from build123d import *

# Parameters (mm, degrees)
SKETCH1_W           = 44.45
SKETCH1_H           = 19.05
BOSS_EXTRUDE1_DEPTH = 12.7
SKETCH2_W           = 7.62
SKETCH2_H           = 16.51
CUT_EXTRUDE1_DEPTH  = 12.7
FILLET1_R           = 1.27
FILLET2_R           = 1.27
SKETCH3_R           = 1.6256
CUT_EXTRUDE2_DEPTH  = 12.7
SKETCH4_R           = 1.651
CUT_EXTRUDE3_DEPTH  = 12.7


with BuildPart() as part:
    # Sketch1 → Boss-Extrude1 (new body)
    with BuildSketch(Plane.XY):
        Rectangle(SKETCH1_W, SKETCH1_H)
    extrude(amount=BOSS_EXTRUDE1_DEPTH)

    # Sketch2 → Cut-Extrude1 (cut)
    with BuildSketch(Plane.XY.offset(12.7)):
        with Locations((-18.415, 1.27)):
            Rectangle(SKETCH2_W, SKETCH2_H)
        with Locations((18.415, 1.27)):
            Rectangle(SKETCH2_W, SKETCH2_H)
    extrude(amount=-CUT_EXTRUDE1_DEPTH, mode=Mode.SUBTRACT)

    # Fillet1
    fillet1_edges = [part.edges().sort_by_distance(p)[0] for p in [
        (-14.605, -6.985, 6.35),
    ]]
    fillet(fillet1_edges, radius=FILLET1_R)

    # Fillet2
    fillet2_edges = [part.edges().sort_by_distance(p)[0] for p in [
        (14.605, -6.985, 6.35),
    ]]
    fillet(fillet2_edges, radius=FILLET2_R)

    # Sketch3 → Cut-Extrude2 (cut)
    with BuildSketch(Plane(origin=(0, 0, 0), x_dir=(-1, 0, 0), z_dir=(0, 0, -1))):
        with Locations((-9.525, 5.715)):
            Circle(SKETCH3_R)
        with Locations((9.525, 5.715)):
            Circle(SKETCH3_R)
    extrude(amount=-CUT_EXTRUDE2_DEPTH, mode=Mode.SUBTRACT)

    # Sketch4 → Cut-Extrude3 (cut)
    with BuildSketch(Plane(origin=(0, -6.985, 0), x_dir=(1, 0, 0), z_dir=(0, 1, 0))):
        with Locations(Location((19.05, -6.35, 0), (0, 0, 180))):
            Circle(SKETCH4_R)
        with Locations(Location((-19.05, -6.4262, 0), (0, 0, 180))):
            Circle(SKETCH4_R)
    extrude(amount=-CUT_EXTRUDE3_DEPTH, mode=Mode.SUBTRACT)


solid = part.part
The model under review builds one solid part; all positions refer to its coordinate system, in mm. A direction names the side the tool comes from. Round coordinates to 2 decimals unless told otherwise and drop trailing zeros. Order: outer loops, then holes, each group sorted by start corner. A loop starts at its lowest first (then second) coordinate and runs counter-clockwise, first axis right, second up. Notation, with made-up numbers: (49.25, -35.75) -> (99.25, -35.75) arc R27 ccw to (99.25, -9.75) -> close; hole circle Ø8 at (21, -33). An arc over 180 degrees is marked (long way). Write item = value, one per line. Start each with the question number.
Item 1: Consider section C-C on z = 5.75. Write out the cut boundary in (x, y) (3 decimals).
Item 2: Mouldability with a two-part tool opening along X and no side actions: class faces 1 (the face through (14.605, 2, 6)), 2 (the face through (-17.4, -8.2, 6.5)), 3 (the face through (18, -6.985, 8)) as released by +X, released by -X, zero draft, split by the parting line, or undercut.
Item 3: Consider section A-A on x = 19.05. Write out the cut boundary in (y, z) (3 decimals).
Item 4: Clearance check with flat-ended pins moving along their axes: pin 1 Ø4 at (y, z) = (-1.5, 9) entering from -X (3 decimals); pin 2 Ø1.9 at (x, z) = (-20.5, 4) entering from +Y (3 decimals); pin 3 Ø4 at (y, z) = (-2, 6) entering from +X (3 decimals). State where each tip first meets the part, or that it passes through.
Item 5: For faces 4 (the face through (-14.605, 2, 6)), 5 (the face through (22.225, -8, 6)), list the 3-axis set-ups (+Z, -Z, +X, -X, +Y, -Y) from which the entire face can be reached by the end or side of a thin tool; tool diameter is ignored.
Item 6: Consider section B-B on y = 5.25. Write out the cut boundary in (x, z) (3 decimals).
Item 7: For line 1 along Z through (x, y) = (19.05, -8.85); line 2 along X through (y, z) = (6.25, 4) (3 decimals); line 3 along X through (y, z) = (5.5, 9) (3 decimals), list the stretches that pass through material, from the lowest coordinate up.
Item 8: Consider section D-D on z = 1.5. Write out the cut boundary in (x, y) (3 decimals).
Conclusion:
q1.outline = (-22.225, -9.525) -> (-20.556, -9.525) -> (-20.556, -6.985) -> (-22.225, -6.985) -> close; (-17.544, -9.525) -> (17.512, -9.525) -> (17.512, -6.985) -> (15.875, -6.985) arc R1.27 cw to (14.605, -5.715) -> (14.605, 9.525) -> (-14.605, 9.525) -> (-14.605, -5.715) arc R1.27 cw to (-15.875, -6.985) -> (-17.544, -6.985) -> close; (20.588, -9.525) -> (22.225, -9.525) -> (22.225, -6.985) -> (20.588, -6.985) -> close; hole circle Ø3.251 at (-9.525, 5.715); hole circle Ø3.251 at (9.525, 5.715)
q2.face_1 = released by +X
q2.face_2 = undercut
q2.face_3 = zero draft
q3.outline = (-9.525, 0) -> (-6.985, 0) -> (-6.985, 4.699) -> (-9.525, 4.699) -> close; (-9.525, 8.001) -> (-6.985, 8.001) -> (-6.985, 12.7) -> (-9.525, 12.7) -> close
q4.pin_1 = -14.605
q4.pin_2 = -6.985
q4.pin_3 = 14.605
q5.face_4 = +Z, -Z, -X, +Y
q5.face_5 = +Z, -Z, +X, +Y, -Y
q6.outline = (-14.605, 0) -> (-11.083, 0) -> (-11.083, 12.7) -> (-14.605, 12.7) -> close; (-7.967, 0) -> (7.967, 0) -> (7.967, 12.7) -> (-7.967, 12.7) -> close; (11.083, 0) -> (14.605, 0) -> (14.605, 12.7) -> (11.083, 12.7) -> close
q7.line_1 = 0 to 4.7, 8 to 12.7
q7.line_2 = -14.605 to -11.06, -7.99 to 7.99, 11.06 to 14.605
q7.line_3 = -14.605 to -11.136, -7.914 to 7.914, 11.136 to 14.605
q8.outline = (-22.225, -9.525) -> (22.225, -9.525) -> (22.225, -6.985) -> (15.875, -6.985) arc R1.27 cw to (14.605, -5.715) -> (14.605, 9.525) -> (-14.605, 9.525) -> (-14.605, -5.715) arc R1.27 cw to (-15.875, -6.985) -> (-22.225, -6.985) -> close; hole circle Ø3.251 at (-9.525, 5.715); hole circle Ø3.251 at (9.525, 5.715)
